Part model, mm, in its own coordinate system. Round coordinates to 2 decimals unless told otherwise and drop trailing zeros. Write each loop counter-clockwise with the first axis right and the second up, starting at its lowest first coordinate (ties: lowest second). Pieces come first, ordered by that corner, then holes. Notation, with made-up numbers: M -31.75,-25 L 15.25,-25 A26 ccw 15.25,10 Z; hole C -10,-33.75 d9. An arc over 180 degrees is marked long. Use a Markdown table: item, result. Add a question column.
1) Slice it at C-C on y = -58. Write the cut outline in (x, z).
2) Drop a flat-ended pin along its axis: P1, Ø3, axis at x = -81.05, y = 66.75, coming from the -Z side. Give the stop position or say it passes through.
3) Wall check: probe 1 along X at (y, z) = (-0.5, 1.85); probe 2 along Y at (x, z) = (82.5, 0.75); probe 3 along X at (y, z) = (-67, 0.8). Give the ranges that are in metal, low to high.
4) Slice it at A-A on z = 1.3. Give the number of separate pieces and of enclosed holes in the cut face, plus the area to 3 significant figures.
5) Slice it at B-B on x = -42. Write the cut outline in (y, z).
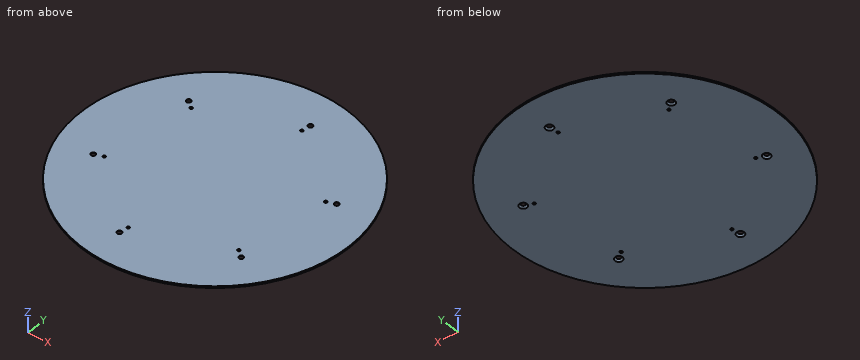
```python
from build123d import *

# Parameters (mm, degrees)
SKETCH1_R                                         = 155
BOSS_EXTRUDE1_DEPTH                               = 2
SKETCH3_R                                         = 1.6
CUT_EXTRUDE2_DEPTH                                = 10
CSK_FOR_8_FLAT_HEAD_MACHINE_SCREW_100_D           = 4.4958
CSK_FOR_8_FLAT_HEAD_MACHINE_SCREW_100_DEPTH       = 10.71
CSK_FOR_8_FLAT_HEAD_MACHINE_SCREW_100_CSINK_D     = 8.780526
CSK_FOR_8_FLAT_HEAD_MACHINE_SCREW_100_CSINK_ANGLE = 82
CSK_FOR_8_FLAT_HEAD_MACHINE_SCREW_100_TIP         = 1.350674586


with BuildPart() as part:
    # Sketch1 → Boss-Extrude1 (new body)
    with BuildSketch(Plane.XY):
        Circle(SKETCH1_R)
    extrude(amount=BOSS_EXTRUDE1_DEPTH)

    # Sketch3 → Cut-Extrude2 (cut)
    with BuildSketch(Plane.XY.offset(2)):
        with Locations((17.280155357, 103.568316733)):
            Circle(SKETCH3_R)
        with Locations((-81.052715639, 66.749211887)):
            Circle(SKETCH3_R)
        with Locations((-98.332870996, -36.819104846)):
            Circle(SKETCH3_R)
        with Locations((-17.280155357, -103.568316733)):
            Circle(SKETCH3_R)
        with Locations((81.052715639, -66.749211887)):
            Circle(SKETCH3_R)
        with Locations((98.332870996, 36.819104846)):
            Circle(SKETCH3_R)
    extrude(amount=-CUT_EXTRUDE2_DEPTH, mode=Mode.SUBTRACT)

    # CSK for #8 Flat Head Machine Screw (100)1
    with Locations(Plane(origin=(0, 0, 0), x_dir=(-1, 0, 0), z_dir=(0, 0, -1))):
        with Locations((-18.981218556, 113.83840056), (89.088513447, 73.366919465), (108.077556089, -40.480982816), (-108.077556089, 40.480982816), (-89.088513447, -73.366919465), (18.981218556, -113.83840056)):
            CounterSinkHole(CSK_FOR_8_FLAT_HEAD_MACHINE_SCREW_100_D / 2, CSK_FOR_8_FLAT_HEAD_MACHINE_SCREW_100_CSINK_D / 2, depth=CSK_FOR_8_FLAT_HEAD_MACHINE_SCREW_100_DEPTH, counter_sink_angle=CSK_FOR_8_FLAT_HEAD_MACHINE_SCREW_100_CSINK_ANGLE)
            with Locations((0, 0, -(CSK_FOR_8_FLAT_HEAD_MACHINE_SCREW_100_DEPTH + CSK_FOR_8_FLAT_HEAD_MACHINE_SCREW_100_TIP / 2))):  # 118° drill point
                Cone(0, CSK_FOR_8_FLAT_HEAD_MACHINE_SCREW_100_D / 2, CSK_FOR_8_FLAT_HEAD_MACHINE_SCREW_100_TIP, mode=Mode.SUBTRACT)


solid = part.part
```
Entries:
| question | item | result |
|---|---|---|
| 1 | outline | M -143.74,0 L 143.74,0 L 143.74,2 L -143.74,2 Z |
| 2 | P1 | passes through |
| 3 | probe 1 | x = -155 to 155 |
| 3 | probe 2 | y = -131.22 to -67.43, -66.07 to 131.22 |
| 3 | probe 3 | x = -139.77 to 79.47, 82.63 to 139.77 |
| 4 | separate pieces | 1 |
| 4 | enclosed holes | 12 |
| 4 | area | 75,200 mm^2 |
| 5 | outline | M -149.2,0 L 149.2,0 L 149.2,2 L -149.2,2 Z |
